CAD build for the part. Positions are in the model's coordinates, mm. A direction names the side the tool comes from. Coordinates: 2 decimals unless noted, no trailing zeros. Order: outer loops, then holes, each group sorted by start corner. A loop starts at its lowest first (then second) coordinate and runs counter-clockwise, first axis right, second up. Notation, with made-up numbers: (-7, 66) - (18, 66) arc R23 ccw to (18, 88) - close; hole circle Ø3 at (51.5, 62.25). An arc over 180 degrees is marked (long way). Use one line per item in the form item = value.
```python
from build123d import *

# Parameters (mm, degrees)
F1_DEPTH  = 2.4
F3_DEPTH  = 2.401
F4_R      = 0.9
F5_DEPTH  = 106.801
F7_DEPTH  = 2.4010001
F9_DEPTH  = 2.4010001
F10_SIZE2 = 1.5
F10_SIZE  = 3
F11_SIZE2 = 3
F11_SIZE  = 1.5
F12_SIZE  = 1
F14_DEPTH = 2.4010001
F15_R     = 2


with BuildPart() as f1:
    # F0 (on Top) → F1 (new body)
    with BuildSketch(Plane.XY):
        Polygon((-10, 86.8), (-10, 61.8), (-4.75, 61.8), (-4.75, 0), (-5.75, 0), (-5.75, -20), (5.75, -20), (5.75, 0), (4.75, 0), (4.75, 61.8), (10, 61.8), (10, 86.8), align=None)
    extrude(amount=F1_DEPTH)

    # F2 (on Top) → F3 (cut, through all)
    with BuildSketch(Plane.XY):
        with BuildLine():
            Line((-3.25, 30), (-3.25, -20))
            Line((-3.25, -20), (2.25, -20))
            Line((2.25, -20), (2.25, -7))
            ThreePointArc((2.25, -7), (1.9571067812, -6.2928932188), (1.25, -6))
            Line((1.25, -6), (0.75, -6))
            ThreePointArc((0.75, -6), (0.0428932188, -5.7071067812), (-0.25, -5))
            Line((-0.25, -5), (-0.25, 30))
            ThreePointArc((-0.25, 30), (-1.75, 31.5), (-3.25, 30))
        make_face()
    extrude(amount=F3_DEPTH, mode=Mode.SUBTRACT)

    # F4 (on face) → F5 (cut, through all)
    with BuildSketch(Plane(origin=(0, 86.8, 0), x_dir=(-1, 0, 0), z_dir=(0, 1, 0))):
        with Locations((-2, 1.2)):
            Circle(F4_R)
        with Locations((2, 1.2)):
            Circle(F4_R)
    extrude(amount=-F5_DEPTH, mode=Mode.SUBTRACT)

    # F6 (on face) → F7 (cut, through all)
    with BuildSketch(Plane.XY.offset(2.4)):
        with BuildLine():
            Line((1, 23.2), (1, 3.2))
            ThreePointArc((1, 3.2), (2, 2.2), (3, 3.2))
            Line((3, 3.2), (3, 23.2))
            ThreePointArc((3, 23.2), (2, 24.2), (1, 23.2))
        make_face()
    extrude(amount=-F7_DEPTH, mode=Mode.SUBTRACT)

    # F8 (on face) → F9 (cut, through all)
    with BuildSketch(Plane.XY.offset(2.4)):
        with BuildLine():
            ThreePointArc((-1, 58.6), (-2, 59.6), (-3, 58.6))
            Line((-3, 58.6), (-3, 38.6))
            ThreePointArc((-3, 38.6), (-2, 37.6), (-1, 38.6))
            Line((-1, 38.6), (-1, 58.6))
        make_face()
    extrude(amount=-F9_DEPTH, mode=Mode.SUBTRACT)

    # F10
    f10_edges = [f1.edges().sort_by_distance(p)[0] for p in [
        (5.75, -20, 1.2),
    ]]
    f10_side = f1.faces().sort_by_distance((5.75, -10, 1.2))[0]
    chamfer(f10_edges, length=F10_SIZE, length2=F10_SIZE2, reference=f10_side)

    # F11
    f11_edges = [f1.edges().sort_by_distance(p)[0] for p in [
        (-5.75, -20, 1.2),
    ]]
    f11_side = f1.faces().sort_by_distance((-4.5, -20, 1.2))[0]
    chamfer(f11_edges, length=F11_SIZE, length2=F11_SIZE2, reference=f11_side)

    # F12
    f12_edges = [f1.edges().sort_by_distance(p)[0] for p in [
        (-3.75, -20, 2.4),
        (-3.75, -20, 0),
        (3.25, -20, 2.4),
        (3.25, -20, 0),
    ]]
    chamfer(f12_edges, length=F12_SIZE)

    # F13 (on face) → F14 (cut, through all)
    with BuildSketch(Plane.XY.offset(2.4)):
        with BuildLine():
            Line((10, 65.6397459622), (10, 82.9602540378))
            ThreePointArc((10, 82.9602540378), (5, 74.3), (10, 65.6397459622))
        make_face()
        with BuildLine():
            Line((-10, 82.9602540378), (-10, 65.6397459622))
            ThreePointArc((-10, 65.6397459622), (-5, 74.3), (-10, 82.9602540378))
        make_face()
    extrude(amount=-F14_DEPTH, mode=Mode.SUBTRACT)

    # F15
    f15_edges = [f1.edges().sort_by_distance(p)[0] for p in [
        (10, 82.960254, 1.2),
        (10, 65.639746, 1.2),
        (10, 86.8, 1.2),
        (-10, 65.639746, 1.2),
        (-10, 82.960254, 1.2),
        (-10, 86.8, 1.2),
    ]]
    fillet(f15_edges, radius=F15_R)


solid = f1.part
```
Item 1: Cut at C-C, the plane y = 72. Write the cut outline in (x, z), plus the area to 3 significant figures.
Derived:
outline = (-5.27, 0) - (5.27, 0) - (5.27, 2.4) - (-5.27, 2.4) - close; hole circle Ø1.8 at (-2, 1.2); hole circle Ø1.8 at (2, 1.2)
area = 20.2 mm²
Item 2: Drill centre lines: line 1 (X direction, y = 24.5, z = 1.15); line 2 (X direction, y = 60.5, z = 1.2); line 3 (Z direction, x = -2, y = 73.75). Where is each one in solid material? Low to high. Write a range as [from, to].
Derived:
line_1 = [-4.75, -3.25], [-0.25, 1.1], [2.9, 4.75]
line_2 = [-4.75, -2.9], [-1.1, 1.1], [2.9, 4.75]
line_3 = [0, 0.3], [2.1, 2.4]
Item 3: Cut at A-A, the plane y = 22. Write the cut outline in (x, z).
Derived:
outline = (-4.75, 0) - (-3.25, 0) - (-3.25, 2.4) - (-4.75, 2.4) - close; (-0.25, 0) - (1, 0) - (1, 2.4) - (-0.25, 2.4) - close; (3, 0) - (4.75, 0) - (4.75, 2.4) - (3, 2.4) - close
Item 4: Drop flat-ended pins along their axis: pin 1 (1.2 mm diameter, centred on y = 11.5, z = 1.5, fed in from -X); pin 2 (1.4 mm diameter, centred on x = -2, z = 1.2, fed in from +Y); pin 3 (0.7 mm diameter, centred on y = 8, z = 1.5, fed in from +X); pin 4 (0.6 mm diameter, centred on x = 1, z = 1, fed in from -Y). Give the stop position or say it passes through.
Derived:
pin_1 = -4.75
pin_2 = through
pin_3 = 4.75
pin_4 = -6
Item 5: Cut at B-B, the plane y = 36.5. Write the cut outline in (x, z), plus the area to 3 significant figures.
Derived:
outline = (-4.75, 0) - (4.75, 0) - (4.75, 2.4) - (-4.75, 2.4) - close; hole circle Ø1.8 at (-2, 1.2); hole circle Ø1.8 at (2, 1.2)
area = 17.7 mm²
Item 6: 3-axis set-ups, long thin cutter, end or side, ignore diameter. For faces 4 (the face through (-7, 61.8, 1)), 5 (the face through (-3.25, 5, 1)), 6 (the face through (1.123, 2.719, 1.75)), 7 (the face through (-5.75, -8, 1)): which of +Z, -Z, +X, -X, +Y, -Y reach the whole face in a straight line?
Derived:
face_4 = +Z, -Z, -X
face_5 = +Z, -Z, -Y
face_6 = +Z, -Z
face_7 = +Z, -Z, -X, -Y
Item 7: Two-plate mould, pull along X, no slides. Class faces 1 (the face through (5.156, -18.188, 1.183)), 2 (the face through (-9.43, 86.2, 1.22)), 3 (the face through (-2.86, 34.61, 1.47)): +X half, -X half, draft (parallel to the pull), parting line (faces both ways), or undercut.
Derived:
face_1 = +X half
face_2 = -X half
face_3 = undercut
